Geometry check sheet. Reference: the model listing, model coordinates, mm. Coordinates: 2 decimals unless noted, no trailing zeros. Order: outer loops, then holes, each group sorted by start corner. A loop starts at its lowest first (then second) coordinate and runs counter-clockwise, first axis right, second up. Notation, with made-up numbers: M 69,74 L 112,74 A24 ccw 112,111 Z; hole C 86.5,-4.5 d1. An arc over 180 degrees is marked long. One line per item, written item: value. Start each with the question number.
1) Sectioned sample at C-C, the plane y = -6.75. Enter the section's corners in (x, z).
2) Sectioned sample at B-B, the plane z = 0. Enter the section's corners in (x, y).
3) Sectioned sample at A-A, the plane x = 0. Enter the section's corners in (y, z), then the cut area to 3 significant figures.
4) Draft check along Z on faces 1 (the cylindrical face through (2.681, 7.489, -6.466)), 2 (the cylindrical face through (-0.54, -9.94, 2.44)). Enter one of: pulls with the +Z half, pulls with the -Z half, needs draft (parallel to the pull), parting line crosses it, or undercut.
5) Go/stop test with flat-tipped pins: P1, Ø6, axis at y = 2, z = -2.5, coming from the +X side; P2, Ø6, axis at x = 0, z = 0, coming from the +Y side; P3, Ø5, axis at y = 4.5, z = 6, coming from the -X side; P4, Ø6, axis at x = -1, z = 4, coming from the +Y side. Record where each tip stops, or that it passes through.
6) Thickness scan on L1, parallel to Y at x = -7.5, z = -3.75; L2, parallel to X at y = -0.5, z = 8.5; L3, parallel to X at y = 4, z = -2.25. Record the ranges inside material, lowest first. Write a range as from..to.
7) Sectioned sample at D-D, the plane x = -5.75. Enter the section's corners in (y, z).
```python
from build123d import *

# Parameters (mm, degrees)
SKETCH_2_R          = 7
CUT_EXTRUDE_1_DEPTH = 10
SKETCH_5_R          = 2.5
CUT_EXTRUDE_3_DEPTH = 10
CUT_EXTRUDE_START   = -10
SKETCH_6_R          = 2.5
CUT_EXTRUDE_4_DEPTH = 10


with BuildPart() as part:
    # 草图1 → 旋转1 (revolve)
    with BuildSketch(Plane.XY):
        with BuildLine():
            Line((0, -10.5), (0, -10))
            ThreePointArc((0, -10), (10, 0), (0, 10))
            Line((0, 10), (0, 10.5))
            ThreePointArc((0, 10.5), (10.5, 0), (0, -10.5))
        make_face()
    revolve(axis=Axis((0, 10, 0), (0, 1, 0)))

    # 草图2 → 切除-拉伸1 (cut)
    with BuildSketch(Plane(origin=(0, 10.5, 0), x_dir=(1, 0, 0), z_dir=(0, 1, 0))):
        with Locations(Location((0, 0, 0), (0, 0, 90))):
            Circle(SKETCH_2_R)
    extrude(amount=-CUT_EXTRUDE_1_DEPTH, mode=Mode.SUBTRACT)

    # 草图5 → 切除-拉伸3 (cut)
    with BuildSketch(Plane(origin=(0, -9.933965028, 0), x_dir=(1, 0, 0), z_dir=(0, 1, 0))):
        Circle(SKETCH_5_R)
    extrude(amount=CUT_EXTRUDE_3_DEPTH, mode=Mode.SUBTRACT)

    # 草图6 → 切除-拉伸4 (cut)
    with BuildSketch(Plane(origin=(0, -9.933965028, 0), x_dir=(1, 0, 0), z_dir=(0, 1, 0)).offset(CUT_EXTRUDE_START)):
        Circle(SKETCH_6_R)
    extrude(amount=CUT_EXTRUDE_4_DEPTH, mode=Mode.SUBTRACT)


solid = part.part
```
Final values:
1. outline: C 0,0 d16.09; hole C 0,0 d14.76
2. outline: M -7,7.14 L -7,7.83 A10.5 ccw -2.5,-10.2 L -2.5,-9.68 A10 cw Z; M 2.5,-10.2 A10.5 ccw 7,7.83 L 7,7.14 A10 cw 2.5,-9.68 Z
3. outline: M -10.2,-2.5 A10.5 ccw 7.83,-7 L 7.14,-7 A10 cw -9.68,-2.5 Z; M -10.2,2.5 L -9.68,2.5 A10 cw 7.14,7 L 7.83,7 A10.5 ccw Z
3. area: 22.0 mm^2
4. face 1: undercut
4. face 2: undercut
5. P1: stops at x = 10.5
5. P2: stops at y = -9.54
5. P3: stops at x = -9.23
5. P4: stops at y = 7.83
6. L1: y = -6.32..-5.45, 5.45..6.32
6. L2: x = -6.14..-5.24, 5.24..6.14
6. L3: x = -9.44..-8.88, 8.88..9.44
7. outline: M 7.14,-3.99 A8.18 cw long 7.14,3.99 L 7.83,3.99 A8.79 ccw long 7.83,-3.99 Z
